```python
from build123d import *

# Parameters (mm, degrees)
BOSS_EXTRUDE1_DEPTH      = 5
BOSS_EXTRUDE1_DEPTH_BACK = 7
SKETCH3_R                = 20
BOSS_EXTRUDE2_DEPTH      = 5
FILLET1_R                = 0.5
SKETCH6_R                = 3.75
CUT_EXTRUDE1_DEPTH       = 15


with BuildPart() as part:
    # Sketch1 → Boss-Extrude1 (new body, two sides)
    with BuildSketch(Plane.ZY.offset(-66.898173267)) as boss_extrude1_sk:
        Polygon((275.981331654, 12.55), (275.981331654, 0.55), (254.516262845, 0.55), (252.302759373, 0.55), (252.302759373, 12.55), (254.516262845, 12.55), align=None)
    extrude(amount=BOSS_EXTRUDE1_DEPTH)
    extrude(boss_extrude1_sk.sketch, amount=-BOSS_EXTRUDE1_DEPTH_BACK)

    # Sketch3 → Boss-Extrude2 (add)
    with BuildSketch(Plane.XY.offset(275.981331654)):
        with Locations((64.647096069, 10.55)):
            Circle(SKETCH3_R)
    extrude(amount=BOSS_EXTRUDE2_DEPTH)

    # Fillet1
    fillet1_edges = [part.edges().sort_by_distance(p)[0] for p in [
        (67.898173267, 12.55, 275.981331654),
        (67.898173267, 0.55, 275.981331654),
        (73.898173267, 6.55, 275.981331654),
        (61.898173267, 6.55, 275.981331654),
    ]]
    fillet(fillet1_edges, radius=FILLET1_R)

    # Sketch6 → Cut-Extrude1 (cut)
    with BuildSketch(Plane(origin=(0, 0, 252.302759373), x_dir=(-1, 0, 0), z_dir=(0, 0, -1))):
        with Locations((-67.969208633, 7.013446821)):
            Circle(SKETCH6_R)
    extrude(amount=-CUT_EXTRUDE1_DEPTH, mode=Mode.SUBTRACT)


solid = part.part
```
Source: CAD feature listing. Evaluate the final solid. Frame: model axes, mm. A direction names the side the tool comes from. Round coordinates to 2 decimals unless told otherwise and drop trailing zeros. Write each loop counter-clockwise with the first axis right and the second up, starting at its lowest first coordinate (ties: lowest second). Pieces come first, ordered by that corner, then holes. Notation, with made-up numbers: M 19.25,54 L 53.25,54 A21 ccw 53.25,69 Z; hole C 22,-1.75 d1. An arc over 180 degrees is marked long. Answer as a JSON object with one key per item and string values. Group by question number.
(1) Section query C-C on x = 65. Output: boundary loops of the cut face in (y, z), then the cut area to 3 significant figures.
(2) Section query B-B on z = 259. Output: boundary loops of the cut face in (x, y).
(3) Section query D-D on z = 271. Output: boundary loops of the cut face in (x, y), then the cut area to 3 significant figures.
(4) Reachability of faces 1 (the flat face through (61.898, 7, 264)), 2 (the flat face through (68, 12.55, 264)), 3 (the flat face through (68, 7, 267.303)) from +Z, -Z, +X, -X, +Y, -Y: full face, straight path, thin tool, end or side. Return the list, or none.
(5) Ray query, line 1 (Y direction, x = 68, z = 259.5); line 2 (Z direction, x = 68.5, y = 9); line 3 (Z direction, x = 80, y = 0.5). Return the intervals inside material, ascending. Write a range as [from, to].
(6) Section query A-A on y = 2.5. Output: boundary loops of the cut face in (x, z), then the cut area to 3 significant figures.
(7) First-contact query: pin 1 (1.5 mm diameter, centred on y = 4, z = 257, fed in from -X); pin 2 (2 mm diameter, centred on x = 74, z = 277, fed in from +Y); pin 3 (3.5 mm diameter, centred on y = 7.5, z = 265.5, fed in from +X). Flat tips, straight axial feed; report the tip coordinate or a pass-through.
(8) Mould query, pull axis Y, two halves, no side actions, for faces 4 (the cylindrical face through (64.505, 5.577, 259.698)), 5 (the flat face through (73.898, 7, 264)), 6 (the flat face through (68, 0.55, 264)). Classes: +Y half, -Y half, draft (parallel to the pull), parting line (faces both ways), or undercut.
Computed values:
{
 "1": {"outline": "M -9.45,275.98 L 0.05,275.98 A0.5 cw 0.55,275.48 L 0.55,252.3 L 4.72,252.3 L 4.72,267.3 L 9.3,267.3 L 9.3,252.3 L 12.55,252.3 L 12.55,275.48 A0.5 cw 13.05,275.98 L 30.55,275.98 L 30.55,280.98 L -9.45,280.98 Z", "area": "416 mm^2"},
 "2": {"outline": "M 61.9,0.55 L 73.9,0.55 L 73.9,12.55 L 61.9,12.55 Z; hole C 67.97,7.01 d7.5"},
 "3": {"outline": "M 61.9,0.55 L 73.9,0.55 L 73.9,12.55 L 61.9,12.55 Z", "area": "144 mm^2"},
 "4": {"face 1": "-Z, -X, +Y, -Y", "face 2": "-Z, +X, -X, +Y", "face 3": "-Z"},
 "5": {"line 1": "[0.55, 3.26], [10.76, 12.55]", "line 2": "[267.3, 280.98]", "line 3": "[275.98, 280.98]"},
 "6": {"outline": "M 46.34,275.98 L 61.4,275.98 A0.5 cw 61.9,275.48 L 61.9,252.3 L 73.9,252.3 L 73.9,275.48 A0.5 cw 74.4,275.98 L 82.96,275.98 L 82.96,280.98 L 46.34,280.98 Z", "area": "467 mm^2"},
 "7": {"pin 1": "x = 61.9", "pin 2": "y = 28.72", "pin 3": "x = 73.9"},
 "8": {"face 4": "undercut", "face 5": "draft", "face 6": "-Y half"}
}
